Source: CAD feature listing. Evaluate the final solid. Frame: model axes, mm. Face numbers are marked on the shaded views. A direction names the side the tool comes from. Give positions to 0.01 mm unless a question says otherwise; leave off trailing zeros. Loops run counter-clockwise (first coordinate to the right, second up) from the corner with the lowest first, then second, coordinate; pieces in that order, holes last. Notation, with made-up numbers: M -11,81 L -4,81 A21 ccw -4,107 Z; hole C 46,35 d11. An arc over 180 degrees is marked long. Answer in a Markdown table with one row per item.
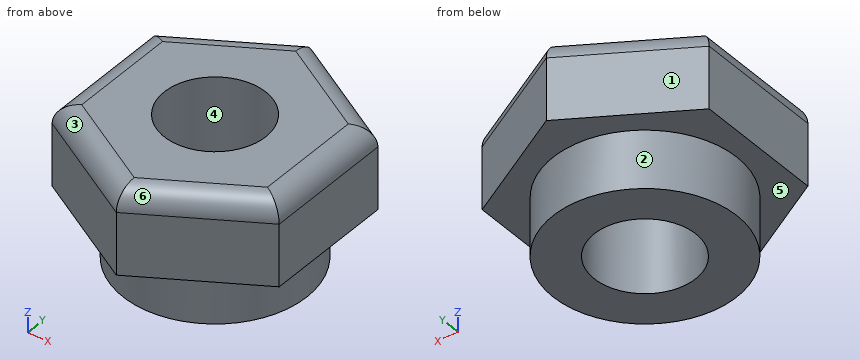
Autodesk Inventor part; units mm, degrees
ref_plane "YZ Plane" through (0, 0, 0) normal (1, 0, 0) x (0, 1, 0)
ref_plane "XZ Plane" through (0, 0, 0) normal (0, 1, 0) x (-1, 0, 0)
ref_plane "XY Plane" through (0, 0, 0) normal (0, 0, 1) x (1, 0, 0)
sketch "スケッチ1" plane through (0, 0, 0) normal (0, 0, 1) x (1, 0, 0)
  line L0 (0, -3.1754) -> (-2.75, -1.5877)
  line L1 (-2.75, -1.5877) -> (-2.75, 1.5877)
  line L2 (-2.75, 1.5877) -> (0, 3.1754)
  line L3 (0, 3.1754) -> (2.75, 1.5877)
  line L4 (2.75, 1.5877) -> (2.75, -1.5877)
  line L5 (2.75, -1.5877) -> (0, -3.1754)
  point P0 (0, 0)
  point P1 (0, 0)
  dimension "d0" = 5.5
extrude "押し出し1" add sketch "スケッチ1" along normal blind 2
sketch "スケッチ2" plane through (0, 0, 0) normal (0, 0, -1) x (-1, 0, 0)
  circle A0 centre (0, 0) radius 2.225
  dimension "d3" = 4.45
extrude "押し出し2" add sketch "スケッチ2" along normal blind 1.4
sketch "スケッチ3" plane through (0, 0, -1.4) normal (0, 0, -1) x (-1, 0, 0)
  point P0 (0, 0)
hole "穴1" at (0, 0, -1.4) direction (0, 0, 1) diameter 2.459 end through all
fillet "フィレット1" radius 0.5 6 edges at (1.375, 2.3816, 2) (2.75, 0, 2) (1.375, -2.3816, 2) (-1.375, -2.3816, 2) (-2.75, 0, 2) (-1.375, 2.3816, 2)
properties part number "BOB-M3-2-3W"
1) Pull-direction query (Y, two-part tool) for the marked faces 1, 2, 3 and 4; classes: released by +Y, released by -Y, zero draft, split by the parting line, or undercut.
Reply:
| item | result |
|---|---|
| face 1 | released by +Y |
| face 2 | split by the parting line |
| face 3 | released by -Y |
| face 4 | undercut |
2) Set-up query: the marked faces 5 and 6. Return all of +Z, -Z, +X, -X, +Y, -Y with unobstructed straight access to the full face (end or side cutting, diameter ignored); none if empty.
Reply:
| item | result |
|---|---|
| face 5 | -Z |
| face 6 | +Z, +X, -Y |
3) Section B-B, the plane z = 0.2. Return loops of the section in (x, y).
Reply:
| item | result |
|---|---|
| outline | M -2.75,-1.59 L 0,-3.18 L 2.75,-1.59 L 2.75,1.59 L 0,3.18 L -2.75,1.59 Z; hole C 0,0 d2.46 |
4) Material intervals for L1, parallel to Y at x = 0, z = -0.45 (1 decimal); L2, parallel to X at y = 0, z = 1.3; L3, parallel to Z at x = 0.7, y = 2.25, sorted ascending.
Reply:
| item | result |
|---|---|
| L1 | y = -2.2 to -1.2, 1.2 to 2.2 |
| L2 | x = -2.75 to -1.23, 1.23 to 2.75 |
| L3 | z = 0 to 2 |
5) Section C-C, the plane y = 0.75. Return loops of the section in (x, z), then the cut area to 3 significant figures.
Reply:
| item | result |
|---|---|
| outline | M -2.75,0 L -2.09,0 L -2.09,-1.4 L -0.97,-1.4 L -0.97,2 L -2.25,2 A0.5 ccw -2.75,1.5 Z; M 0.97,-1.4 L 2.09,-1.4 L 2.09,0 L 2.75,0 L 2.75,1.5 A0.5 ccw 2.25,2 L 0.97,2 Z |
| area | 10.1 mm² |
